For this review, take the finished solid that the model builds, in its own axes (mm). Face numbers are marked on the shaded views. A direction names the side the tool comes from. Give positions to 0.01 mm unless a question says otherwise; leave off trailing zeros. Loops run counter-clockwise (first coordinate to the right, second up) from the corner with the lowest first, then second, coordinate; pieces in that order, holes last. Notation, with made-up numbers: (77, 8.25) - (87, 8.25) arc R12 cw to (87, 30.25) - close; hole circle Ø4 at (52, -8.5). An arc over 180 degrees is marked (long way). Answer in a Markdown table with one row per item.
Autodesk Inventor part; units mm, degrees
ref_plane "YZ Plane" through (0, 0, 0) normal (1, 0, 0) x (0, 1, 0)
ref_plane "XZ Plane" through (0, 0, 0) normal (0, 1, 0) x (-1, 0, 0)
ref_plane "XY Plane" through (0, 0, 0) normal (0, 0, 1) x (1, 0, 0)
sketch "Sketch1" plane through (0, 0, 0) normal (0, 1, 0) x (-1, 0, 0)
  line L0 (0, 15.4608) -> (12.8016, 15.4608)
  line L1 (12.8016, 15.4608) -> (12.8016, -0.338)
  line L2 (12.8016, -0.338) -> (0, -0.338)
  line L3 (0, -0.338) -> (0, 15.4608)
extrude "Extrusion1" add sketch "Sketch1" along normal blind 12.192
sketch "Sketch2" plane through (-12.8016, 0, 15.4608) normal (0, 0, 1) x (1, 0, 0)
  arc A0 (6.4008, 0) -> (6.4008, 12.192) centre (6.4008, 6.096) ccw
  line L0 (0, 12.192) -> (12.8016, 12.192)
  line L1 (12.8016, 0) -> (0, 0)
  line L2 (6.4008, 0) -> (17.5033, -4.1356)
  line L3 (17.5033, -4.1356) -> (19.4121, 8.0167)
  line L4 (19.4121, 8.0167) -> (11.5072, 13.7088)
  line L5 (11.5072, 13.7088) -> (6.4008, 12.192)
extrude "Extrusion2" cut sketch "Sketch2" along normal mid plane 2540
sketch "Sketch3" plane through (-12.8016, 0, 15.4608) normal (0, 0, 1) x (1, 0, 0)
  arc A0 (6.4008, 0) -> (6.4008, 12.192) centre (6.4008, 6.096) ccw
  circle A1 centre (6.4008, 6.096) radius 2.54
  point P0 (12.8016, 0)
  dimension "d8" = 5.08
extrude "Extrusion3" cut sketch "Sketch3" against normal blind 2540
sketch "Sketch4" plane through (-12.8016, 0, -0.338) normal (-1, 0, 0) x (0, 0, 1)
  circle A0 centre (7.8994, 6.096) radius 7.8994
  point P0 (0.338, 0)
extrude "Extrusion4" add sketch "Sketch4" along normal blind 8.89
sketch "Sketch5" plane through (-21.6916, 6.096, 7.5614) normal (-1, 0, 0) x (0, 0, 1)
  circle A0 centre (0, 0) radius 7.8994
  line L0 (-7.8994, 0) -> (7.8994, 0)
  line L1 (1.5587, -11.4554) -> (1.5587, -7.7441)
  line L2 (-1.5587, -7.7441) -> (-1.5587, -11.4554)
  line L3 (-6.1592, -11.4554) -> (-1.5587, -11.4554)
  line L4 (1.5587, -11.4554) -> (6.1592, -11.4554)
  arc A1 (-6.1592, -11.4554) -> (6.1592, -11.4554) centre (0, -7.8994) ccw
  line L5 (-1.5587, -7.7441) -> (1.5587, -7.7441)
  line L6 (1.5587, 7.7441) -> (-1.5587, 7.7441)
  line L7 (1.5587, 7.7441) -> (1.5587, 11.4554)
  line L8 (-1.5587, 11.4554) -> (-1.5587, 7.7441)
  line L9 (-1.5587, 11.4554) -> (-6.1592, 11.4554)
  arc A2 (6.1592, 11.4554) -> (-6.1592, 11.4554) centre (0, 7.8994) ccw
  line L10 (6.1592, 11.4554) -> (1.5587, 11.4554)
  point P0 (-7.5614, -6.096)
  dimension "d16" = 360
extrude "Extrusion5" add sketch "Sketch5" against normal blind 2.54 contours L6 A0 | A0 L8 L9 A2 L10 L7 | L1 L4 A1 L3 L2 A0
sketch "Sketch6" plane through (-21.6916, 0, -0.338) normal (-1, 0, 0) x (0, 0, 1)
  arc A0 (2.8755, 12.192) -> (0, 6.096) centre (7.8994, 6.096) ccw
  circle A1 centre (7.8994, 6.096) radius 2.54
  point P0 (0.338, 0)
  dimension "d20" = 5.08
extrude "Extrusion6" add sketch "Sketch6" along normal blind 2.54
sketch "Sketch7" plane through (-24.2316, 6.096, 7.5614) normal (-1, 0, 0) x (0, 0, 1)
  circle A0 centre (0, 0) radius 3.175
  point P0 (-7.5614, -6.096)
  dimension "d23" = 6.35
extrude "Extrusion7" add sketch "Sketch7" along normal blind 1.27
sketch "Sketch10" plane through (-25.5016, 6.096, 7.5614) normal (-1, 0, 0) x (0, 0, 1)
  point P0 (-7.5614, -6.096)
properties part number "Germi01-03-01"
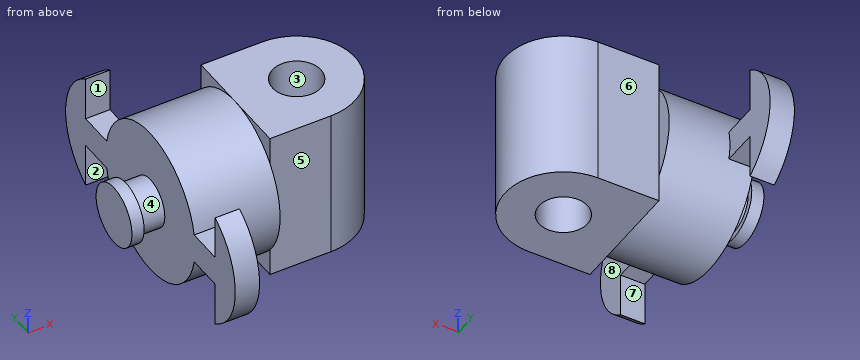
1. Mouldability with a two-part tool opening along Y and no side actions: class the marked faces 6, 7 and 8 as released by +Y, released by -Y, zero draft, split by the parting line, or undercut.
Values:
| item | result |
|---|---|
| face 6 | released by +Y |
| face 7 | undercut |
| face 8 | zero draft |
2. Wall thickness on line 1 (Y direction, x = -12.5, z = 6); line 2 (X direction, y = 13, z = 4); line 3 (X direction, y = 17.5, z = 8.5): over which ranges is each line inside the solid? List them lowest first. Write a range as [from, to].
Values:
| item | result |
|---|---|
| line 1 | y = [0, 12.19] |
| line 2 | x = [-21.69, -12.8] |
| line 3 | x = [-21.69, -19.15] |
3. We need section C-C, the plane x = -4.25. Give the boundary of the cut face in (y, z).
Values:
| item | result |
|---|---|
| outline | (0.39, -0.34) - (4.74, -0.34) - (4.74, 15.46) - (0.39, 15.46) - close; (7.45, -0.34) - (11.8, -0.34) - (11.8, 15.46) - (7.45, 15.46) - close |
4. For the marked faces 1, 2, 3, 4 and 5, list the 3-axis set-ups (+Z, -Z, +X, -X, +Y, -Y) from which the entire face can be reached by the end or side of a thin tool; tool diameter is ignored.
Values:
| item | result |
|---|---|
| face 1 | +Z, +X, -X |
| face 2 | -Z, +X, -X |
| face 3 | +Z, -Z |
| face 4 | none |
| face 5 | +Z, -Z, +X, -Y |
5. Clearance check with flat-ended pins moving along their axes: pin 1 (1.3 mm diameter, centred on x = -21, z = 12.5, fed in from +Y); pin 2 (8 mm diameter, centred on x = -16.5, z = 7, fed in from -Y); pin 3 (5 mm diameter, centred on x = -9.5, z = 4, fed in from +Y); pin 4 (1.5 mm diameter, centred on x = -20, y = 11, fed in from +Z). State where each tip first meets the part, or that it passes through.
Values:
| item | result |
|---|---|
| pin 1 | stops at y = 19.67 |
| pin 2 | stops at y = -8.92 |
| pin 3 | stops at y = 12.19 |
| pin 4 | stops at z = 14.28 |
